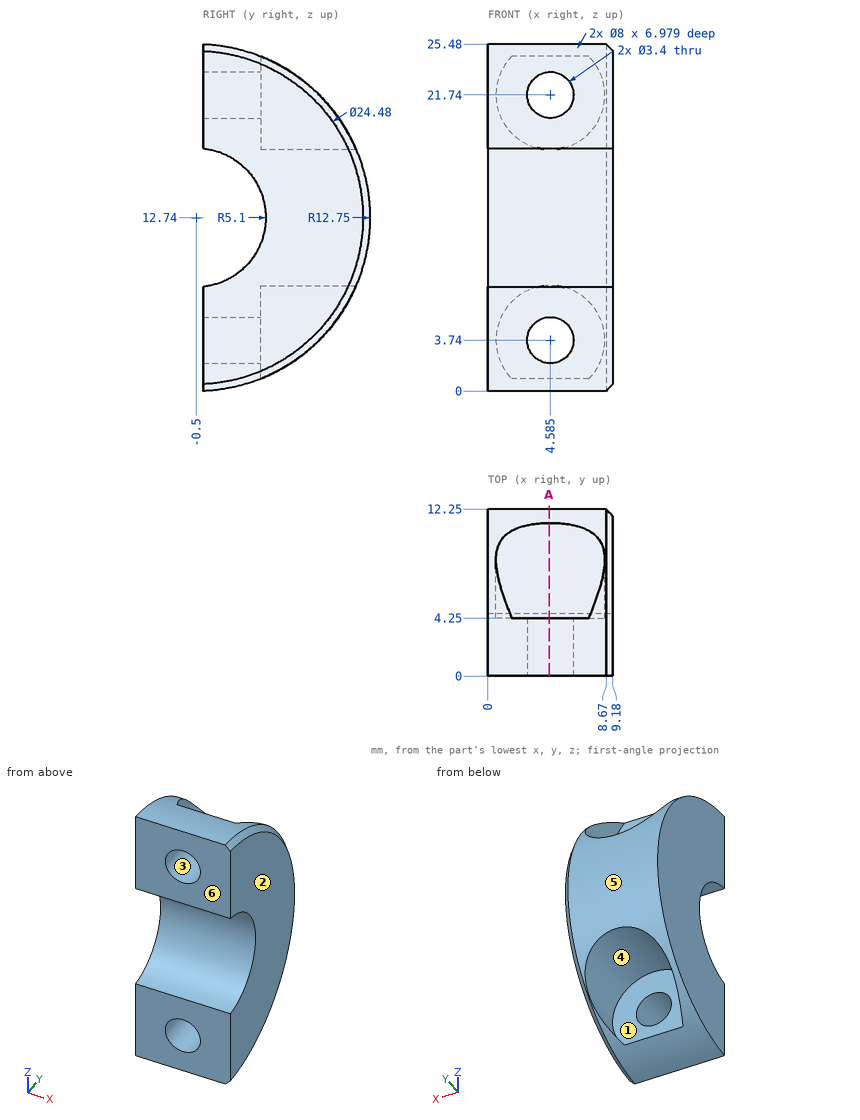
Input: dimensioned drawing with shaded views. Units: mm. Origin: part minimum x, y, z. A direction names the side the tool comes from. Coordinates: 2 decimals unless noted, no trailing zeros. Return JSON: item names as keys, results as strings. Group by question number.
1. Cut plane A-A (x = 4.5). Count the separate pieces of the cut face and the enclosed holes in it.
2. Pull-direction query (Z, two-part tool) for the marked faces 3, 4, 5 and 6; classes: pulls with the +Z half, pulls with the -Z half, needs draft (parallel to the pull), parting line crosses it, or undercut.
3. Pin query (flat end, axial travel): pin 1 (1.5 mm diameter, centred on y = 9.5, z = 4, fed in from -X); pin 2 (4 mm diameter, centred on x = 8, y = 4.5, fed in from +Z); pin 3 (2 mm diameter, centred on x = 4.59, z = 21.74, fed in from +Y); pin 4 (2 mm diameter, centred on x = 5.5, z = 21.5, fed in from +Y). Return the tip coordinate at first contact, or that it passes through.
4. Set-up query: the marked faces 1 and 2. Return all of +Z, -Z, +X, -X, +Y, -Y with unobstructed straight access to the full face (end or side cutting, diameter ignored); none if empty.
5. Material intervals for line 1 along Y through (x, z) = (2.5, 20.75); line 2 along Z through (x, y) = (1.75, 2.75); line 3 along X through (y, z) = (7.25, 22.25), sorted ascending. Write a range as [from, to].
Resolved:
{
 "1": {"separate pieces": "3", "enclosed holes": "0"},
 "2": {"face 3": "undercut", "face 4": "undercut", "face 5": "parting line crosses it", "face 6": "needs draft"},
 "3": {"pin 1": "stops at x = 0", "pin 2": "stops at z = 25.13", "pin 3": "passes through", "pin 4": "stops at y = 4.25"},
 "4": {"face 1": "+Y", "face 2": "+Z, -Z, +X, +Y, -Y"},
 "5": {"line 1": "y = [0, 4.25]", "line 2": "z = [0.41, 8.81], [16.67, 25.07]", "line 3": "x = [0, 0.62], [8.55, 9.15]"}
}
